Here's how the part is built. I have some questions about the finished solid (model axes, mm). Face numbers are marked on the shaded views. A direction names the side the tool comes from. Round coordinates to 2 decimals unless told otherwise and drop trailing zeros. Order: outer loops, then holes, each group sorted by start corner. A loop starts at its lowest first (then second) coordinate and runs counter-clockwise, first axis right, second up. Notation, with made-up numbers: (-19, 3.5) -> (-13, 3.5) arc R6 ccw to (-13, 9.5) -> close; hole circle Ø7 at (78.25, 13.5). An arc over 180 degrees is marked (long way). One line per item, written item: value.
```python
from build123d import *

# Parameters (mm, degrees)
F0_W     = 5
F0_H     = 18.05
F0_W_2   = 20
F1_DEPTH = 2.5
F2_DEPTH = 15
F4_DEPTH = 30.001


with BuildPart() as f1:
    # F0 (on Top) → F1 (new body)
    with BuildSketch(Plane.XY):
        with Locations((2.5, 9.025)):
            Rectangle(F0_W, F0_H)
        with Locations((15, 9.025)):
            Rectangle(F0_W_2, F0_H)
        with Locations((27.5, 9.025)):
            Rectangle(F0_W, F0_H)
    extrude(amount=-F1_DEPTH)

    # F0 (on Top) → F2 (join)
    with BuildSketch(Plane.XY):
        with Locations((2.5, 9.025)):
            Rectangle(F0_W, F0_H)
        with Locations((27.5, 9.025)):
            Rectangle(F0_W, F0_H)
    extrude(amount=F2_DEPTH)

    # F3 (on face) → F4 (cut, through all)
    with BuildSketch(Plane.YZ.offset(30)):
        with BuildLine():
            ThreePointArc((4.025, 15), (9.025, 10), (14.025, 15))
            Line((14.025, 15), (4.025, 15))
        make_face()
        with BuildLine():
            Line((4.025, 15), (14.025, 15))
            ThreePointArc((14.025, 15), (9.025, 20), (4.025, 15))
        make_face()
    extrude(amount=-F4_DEPTH, mode=Mode.SUBTRACT)


solid = f1.part
```
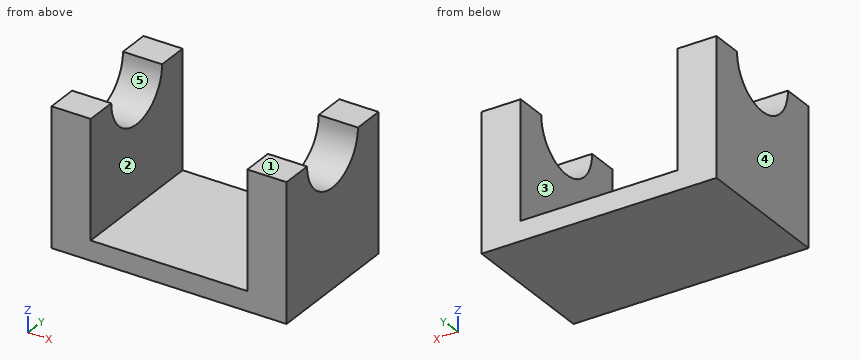
Q1. I need wall thicknesses on line 1 along X through (y, z) = (8, 8); line 2 along Z through (x, y) = (19.5, 8.5); line 3 along Y through (x, z) = (28.5, 11.5). Which ranges of each line are inside material? Lowest first, please.
Answers:
line 1: 0 to 5, 25 to 30
line 2: -2.5 to 0
line 3: 0 to 5.45, 12.6 to 18.05
Q2. I want a section at B-B on y = 1.5. Write out the boundary of the cut face in (x, z).
Answers:
outline: (0, -2.5) -> (30, -2.5) -> (30, 15) -> (25, 15) -> (25, 0) -> (5, 0) -> (5, 15) -> (0, 15) -> close
Q3. If we mould it in two halves opening along X, with no side actions, what happens to the marked faces 3, 4 and 5? For each: pulls with the +X half, pulls with the -X half, needs draft (parallel to the pull), parting line crosses it, or undercut.
Answers:
face 3: undercut
face 4: pulls with the -X half
face 5: needs draft
Q4. For P1, Ø8, axis at x = 17.5, y = 4.5, coming from the +Z side; P2, Ø4, axis at x = 4.5, y = 11.5, coming from the +Z side, each with a flat end and sliding along its axis, tell me the tip position at first contact or that it passes through.
Answers:
P1: z = 0
P2: z = 12.77
Q5. I want a section at A-A on z = 3.5. Write out the boundary of the cut face in (x, y).
Answers:
outline: (0, 0) -> (5, 0) -> (5, 18.05) -> (0, 18.05) -> close; (25, 0) -> (30, 0) -> (30, 18.05) -> (25, 18.05) -> close
Q6. I want a section at D-D on x = 26. Write out the boundary of the cut face in (y, z) (3 decimals), then the cut area to 3 significant figures.
Answers:
outline: (0, -2.5) -> (18.05, -2.5) -> (18.05, 15) -> (14.025, 15) arc R5 cw to (4.025, 15) -> (0, 15) -> close
area: 277 mm2
Q7. Which directions (+Z, -Z, +X, -X, +Y, -Y) give clear straight access to the entire face, cutting with the end or side of a thin tool? Please do the marked faces 1 and 2.
Answers:
face 1: +Z, +X, -X, +Y, -Y
face 2: +Z, +Y, -Y
Q8. I want a section at C-C on z = 11. Write out the boundary of the cut face in (x, y) (3 decimals), then the cut area to 4 significant figures.
Answers:
outline: (0, 0) -> (5, 0) -> (5, 6.025) -> (0, 6.025) -> close; (0, 12.025) -> (5, 12.025) -> (5, 18.05) -> (0, 18.05) -> close; (25, 0) -> (30, 0) -> (30, 6.025) -> (25, 6.025) -> close; (25, 12.025) -> (30, 12.025) -> (30, 18.05) -> (25, 18.05) -> close
area: 120.5 mm2
